Geometry check sheet. Reference: the model listing, model coordinates, mm. Face numbers are marked on the shaded views. A direction names the side the tool comes from. Give positions to 0.01 mm unless a question says otherwise; leave off trailing zeros. Write each loop counter-clockwise with the first axis right and the second up, starting at its lowest first coordinate (ties: lowest second). Pieces come first, ordered by that corner, then holes.
(1) Depth check by flat-ended pin: P1, Ø1.5, axis at y = 15, z = 17.5, coming from the -X side; P2, Ø8, axis at x = 8.5, z = -19, coming from the +Y side; P3, Ø2.5, axis at x = 0.5, z = 16, coming from the +Y side; P4, Ø10, axis at y = 38.5, z = -12.5, coming from the +X side. Enter the tip coordinate at first touch or a pass-through.
(2) Cross-section at C-C (z = 17.5). Record the boundary of the cut face in (x, y).
(3) Thickness scan on line 1 along X through (y, z) = (24.5, 0); line 2 along X through (y, z) = (16, 0); line 3 along Y through (x, z) = (-3, -8). Record the ranges inside material, lowest first.
(4) Mould release check, pull along X, two halves, no side actions. Record for the marked faces 3, 4 and 5: +X half, -X half, draft (parallel to the pull), parting line (faces both ways), or undercut.
(5) Cross-section at D-D (y = 29). Record the boundary of the cut face in (x, z).
(6) Tool access check on the marked faces 1 and 2. Record the directions out of +Z, -Z, +X, -X, +Y, -Y that give a thin tool (end or side, any length) a straight path to the whole face; none if there is none.
(7) Cross-section at A-A (x = 0). Record the boundary of the cut face in (y, z), and give its area (3 significant figures).
(8) Cross-section at B-B (y = 18.5). Record the boundary of the cut face in (x, z), and give its area (3 significant figures).
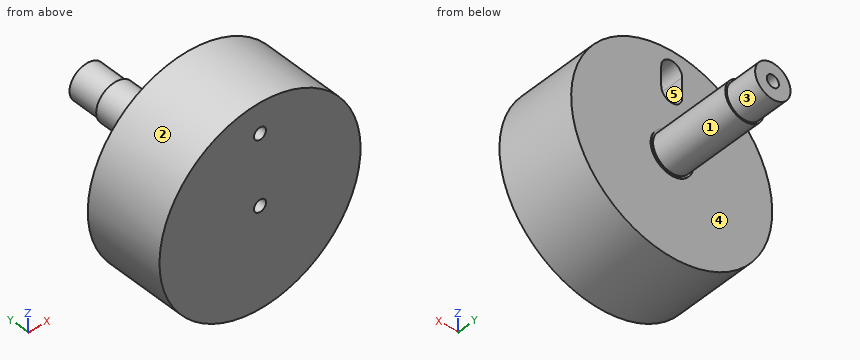
```python
from build123d import *

# Parameters (mm, degrees)
SKETCH1_R           = 25
BOSS_EXTRUDE1_DEPTH = 20
CUT_EXTRUDE2_DEPTH  = 10
SKETCH5_R           = 1.5
CUT_EXTRUDE3_DEPTH  = 37.742346142
SKETCH2_R           = 5.25
BOSS_EXTRUDE2_DEPTH = 0.2
SKETCH7_R           = 4.8
BOSS_EXTRUDE3_DEPTH = 20.1
SKETCH8_R           = 4.4
BOSS_EXTRUDE4_DEPTH = 7.9
SKETCH6_R           = 1.5
CUT_EXTRUDE4_DEPTH  = 60.776584044


with BuildPart() as part:
    # Sketch1 → Boss-Extrude1 (new body)
    with BuildSketch(Plane(origin=(0, 0, 0), x_dir=(1, 0, 0), z_dir=(0, 1, 0))):
        with Locations(Location((0, 0, 0), (0, 0, 270))):
            Circle(SKETCH1_R)
    extrude(amount=BOSS_EXTRUDE1_DEPTH)

    # Sketch3 → Cut-Extrude2 (cut)
    with BuildSketch(Plane(origin=(0, 20, 0), x_dir=(1, 0, 0), z_dir=(0, 1, 0))):
        with BuildLine():
            Line((-2.6, -15), (-2.6, -20))
            ThreePointArc((-2.6, -20), (0, -22.6), (2.6, -20))
            Line((2.6, -20), (2.6, -15))
            ThreePointArc((2.6, -15), (0, -12.4), (-2.6, -15))
        make_face()
    extrude(amount=-CUT_EXTRUDE2_DEPTH, mode=Mode.SUBTRACT)

    # Sketch5 → Cut-Extrude3 (cut, through all)
    with BuildSketch(Plane(origin=(0, 10, 0), x_dir=(1, 0, 0), z_dir=(0, 1, 0))):
        with Locations(Location((0, -17.5, 0), (0, 0, 270))):
            Circle(SKETCH5_R)
    extrude(amount=-CUT_EXTRUDE3_DEPTH, mode=Mode.SUBTRACT)

    # Sketch2 → Boss-Extrude2 (add)
    with BuildSketch(Plane(origin=(0, 20, 0), x_dir=(1, 0, 0), z_dir=(0, 1, 0))):
        with Locations(Location((0, 0, 0), (0, 0, 270))):
            Circle(SKETCH2_R)
    extrude(amount=BOSS_EXTRUDE2_DEPTH)

    # Sketch7 → Boss-Extrude3 (add)
    with BuildSketch(Plane(origin=(0, 20.2, 0), x_dir=(1, 0, 0), z_dir=(0, 1, 0))):
        with Locations(Location((0, 0, 0), (0, 0, 270))):
            Circle(SKETCH7_R)
    extrude(amount=BOSS_EXTRUDE3_DEPTH)

    # Sketch8 → Boss-Extrude4 (add)
    with BuildSketch(Plane(origin=(0, 40.3, 0), x_dir=(1, 0, 0), z_dir=(0, 1, 0))):
        with Locations(Location((0, 0, 0), (0, 0, 270))):
            Circle(SKETCH8_R)
    extrude(amount=BOSS_EXTRUDE4_DEPTH)

    # Sketch6 → Cut-Extrude4 (cut, through all)
    with BuildSketch(Plane.XZ):
        with Locations(Location((0, 0, 0), (0, 0, 270))):
            Circle(SKETCH6_R)
    extrude(amount=-CUT_EXTRUDE4_DEPTH, mode=Mode.SUBTRACT)


solid = part.part
```
Reply:
1. P1: stops at x = -18.56
1. P2: stops at y = 20
1. P3: stops at y = 10
1. P4: passes through
2. outline: (-17.85, 0) - (-1.5, 0) - (-1.5, 10) - (-2.6, 10) - (-2.6, 20) - (-17.85, 20) - close; (1.5, 0) - (17.85, 0) - (17.85, 20) - (2.6, 20) - (2.6, 10) - (1.5, 10) - close
3. line 1: x = -4.8 to -1.5, 1.5 to 4.8
3. line 2: x = -25 to -1.5, 1.5 to 25
3. line 3: y = 0 to 20
4. face 3: parting line
4. face 4: draft
4. face 5: undercut
5. outline: circle Ø9.6 at (0, 0); hole circle Ø3 at (0, 0)
6. face 1: +Y
6. face 2: +Y, -Y
7. outline: (0, -25) - (20, -25) - (20, -5.25) - (20.2, -5.25) - (20.2, -4.8) - (40.3, -4.8) - (40.3, -4.4) - (48.2, -4.4) - (48.2, -1.5) - (0, -1.5) - close; (0, 1.5) - (48.2, 1.5) - (48.2, 4.4) - (40.3, 4.4) - (40.3, 4.8) - (20.2, 4.8) - (20.2, 5.25) - (20, 5.25) - (20, 12.4) - (10, 12.4) - (10, 16) - (0, 16) - close; (0, 19) - (10, 19) - (10, 22.6) - (20, 22.6) - (20, 25) - (0, 25) - close
7. area: 988 mm2
8. outline: circle Ø50 at (0, 0); hole (-2.6, 15) arc R2.6 ccw to (2.6, 15) - (2.6, 20) arc R2.6 ccw to (-2.6, 20) - close; hole circle Ø3 at (0, 0)
8. area: 1,910 mm2
